Here's how the part is built. I have some questions about the finished solid (model axes, mm). Give positions to 0.01 mm unless a question says otherwise; leave off trailing zeros. Loops run counter-clockwise (first coordinate to the right, second up) from the corner with the lowest first, then second, coordinate; pieces in that order, holes last.
Q1. If we section it at B-B (y = 55): Please give me the cut outline in (x, z).
Q2. Will these pins go through, and if not, where does the flat tip stop? P1, Ø7, axis at x = -3, z = 0, coming from the +Y side; P2, Ø6, axis at x = 7.5, y = -7.5, coming from the -Z side; P3, Ø3, axis at y = -6.5, z = 7, coming from the +X side; P4, Ø5, axis at x = -5.5, y = 49, coming from the -Z side.
Q3. If we section it at A-A (y = 88.5): Please give me the cut outline in (x, z).
Q4. I need wall thicknesses on line 1 (X direction, y = -8.25, z = 0); line 2 (X direction, y = 17, z = 0.75). Which ranges of each line are inside material? Lowest first, please.
Autodesk Inventor part; units mm, degrees
ref_plane "YZ Plane" through (0, 0, 0) normal (1, 0, 0) x (0, 1, 0)
ref_plane "XZ Plane" through (0, 0, 0) normal (0, 1, 0) x (-1, 0, 0)
ref_plane "XY Plane" through (0, 0, 0) normal (0, 0, 1) x (1, 0, 0)
sketch "Sketch1" plane through (0, 0, 0) normal (1, 0, 0) x (0, 1, 0)
  line L0 (0, 0) -> (101.6, 0)
  line L1 (0, -11.557) -> (0, -13.462)
  line L2 (0, -13.462) -> (101.6, 0)
  line L3 (0, 0) -> (-25.4, 0)
  line L4 (-25.4, 0) -> (-25.4, -11.557)
  line L5 (-25.4, -11.557) -> (0, -11.557)
  line L6 (1.27, -10.287) -> (1.27, -12.0126)
  line L7 (1.27, -12.0126) -> (82.3464, -1.27)
  line L8 (0, -10.287) -> (-24.13, -10.287)
  line L9 (82.3464, -1.27) -> (91.9313, 0)
  line L10 (0, -10.287) -> (1.27, -10.287)
  line L11 (-24.13, -10.287) -> (-25.4, -10.287)
  dimension "d0" = 101.6
  dimension "d1" = 13.462
  dimension "d2" = 25.4
  dimension "d3" = 11.557
  dimension "d4" = 1.27
  dimension "d5" = 1.27
revolve "Revolution1" add sketch "Sketch1" angle 360 about axis through (0, 0, 0) along (0, 1, 0) contours L0 L2 L1 L5 L4 L11 L8 L10 L6 L7 L9
sketch "Sketch2" plane through (0, -25.4, 0) normal (0, -1, 0) x (1, 0, 0)
  circle A0 centre (0, 0) radius 11.557
  circle A1 centre (0, 0) radius 11.811
  circle A2 centre (0, 0) radius 11.557
  line L0 (-0.0952, -11.5566) -> (-1.6827, -11.5566)
  line L1 (-1.6827, -11.5566) -> (1.4923, -11.5566)
  line L2 (-1.6827, -11.5566) -> (1.4923, -11.5566) construction
  line L3 (0, 0) -> (-15.1978, 0)
  line L4 (-11.557, 0) -> (-11.557, -1.5875)
  line L5 (-11.557, 0) -> (-9.9695, 0) construction
  line L6 (-11.557, 0) -> (-11.557, 1.5875)
  line L7 (-0.0029, 11.557) -> (-1.5904, 11.557)
  line L8 (-0.0029, 11.557) -> (1.5846, 11.557)
  line L9 (11.557, -0.0003) -> (11.557, 1.5872)
  line L10 (11.557, -0.0003) -> (13.1445, -0.0003) construction
  line L11 (11.557, 1.5872) -> (11.557, -1.5806)
  line L12 (1.5846, 11.7042) -> (1.5846, 11.4479)
  line L13 (1.5846, 11.7042) -> (1.8409, 11.7042) construction
  line L14 (-1.5846, 11.7042) -> (-1.5846, 11.4479)
  line L15 (-1.5846, 11.7042) -> (-1.3282, 11.7042) construction
  line L16 (-11.4484, 1.5806) -> (-11.7048, 1.5806)
  line L17 (-11.7048, -1.5806) -> (-11.4474, -1.5882)
  line L18 (11.7048, -1.5806) -> (11.4484, -1.5806)
  circle A3 centre (0, 0) radius 11.557
  circle A4 centre (0, 0) radius 11.811
  line L19 (-11.7042, -1.5846) -> (-11.4479, -1.5846)
  line L20 (-11.7042, -1.5846) -> (-11.7042, -1.3282) construction
  line L21 (-11.557, -0.0029) -> (-11.557, -1.5904)
  line L22 (-11.557, -0.0029) -> (-11.557, 1.5846)
  line L23 (-11.7042, 1.5846) -> (-11.4479, 1.5846)
  line L24 (-11.7042, 1.5846) -> (-11.7042, 1.8409) construction
  circle A5 centre (0, 0) radius 11.557
  circle A6 centre (0, 0) radius 11.811
  line L25 (1.5846, -11.7042) -> (1.5846, -11.4479)
  line L26 (1.5846, -11.7042) -> (1.3282, -11.7042) construction
  line L27 (0.0029, -11.557) -> (1.5904, -11.557)
  line L28 (0.0029, -11.557) -> (-1.5846, -11.557)
  line L29 (-1.5846, -11.7042) -> (-1.5846, -11.4479)
  line L30 (-1.5846, -11.7042) -> (-1.8409, -11.7042) construction
  circle A7 centre (0, 0) radius 11.557
  circle A8 centre (0, 0) radius 11.811
  line L31 (11.7042, 1.5846) -> (11.4479, 1.5846)
  line L32 (11.7042, 1.5846) -> (11.7042, 1.3282) construction
  line L33 (11.557, 0.0029) -> (11.557, 1.5904)
  line L34 (11.557, 0.0029) -> (11.557, -1.5846)
  line L35 (11.7042, -1.5846) -> (11.4479, -1.5846)
  line L36 (11.7042, -1.5846) -> (11.7042, -1.8409) construction
  point P0 (11.5566, -0.0952)
  point P1 (0.0003, 11.557)
  point P2 (-1.5806, -11.4484)
  point P3 (1.5882, -11.4474)
  point P4 (-1.5806, -11.7048)
  point P5 (1.5806, -11.7048)
  point P6 (1.5806, 11.7048)
  point P7 (0.0952, 11.5566)
  point P8 (-11.557, 0.0003)
  point P9 (11.4484, -1.5806)
  point P10 (11.4474, 1.5882)
  point P11 (11.7048, -1.5806)
  point P12 (11.7048, 1.5806)
  point P13 (-11.7048, 1.5806)
  point P14 (-11.5566, 0.0952)
  point P15 (-0.0003, -11.557)
  point P16 (1.5806, 11.4484)
  point P17 (-1.5882, 11.4474)
  point P18 (1.5806, 11.7048)
  point P19 (-1.5806, 11.7048)
  point P20 (-1.5806, -11.7048)
  dimension "d7" = 0.254
  dimension "d8" = 1.5875
  dimension "d9" = 3.175
  dimension "d10" = 0
  dimension "d11" = 1.5875
  dimension "d12" = 90
  dimension "d13" = 1.5875
  dimension "d14" = 1.5875
  dimension "d15" = 1.5875
  dimension "d20" = 90
  dimension "d21" = 90
  dimension "d25" = 360
properties part number "Nose Cone MK II [incomplete]"
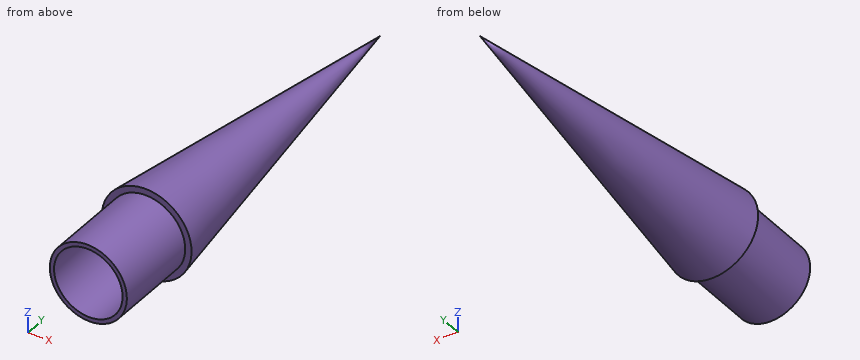
Check sheet entries:
1. outline: circle Ø12.35 at (0, 0); hole circle Ø9.79 at (0, 0)
2. P1: stops at y = 101.6
2. P2: stops at z = -10.64
2. P3: stops at x = 10.16
2. P4: stops at z = -6.35
3. outline: circle Ø3.47 at (0, 0); hole circle Ø0.91 at (0, 0)
4. line 1: x = -11.56 to -10.29, 10.29 to 11.56
4. line 2: x = -11.18 to -9.9, 9.9 to 11.18
